from build123d import *

# Parameters (mm, degrees)
F0_W     = 3.9
F0_H     = 3.5
F1_DEPTH = 0.7
F3_DEPTH = 1
F4_SIZE  = 0.3
F6_DEPTH = 0.7


with BuildPart() as f1:
    # F0 (on Right) → F1 (new body)
    with BuildSketch(Plane.YZ):
        Rectangle(F0_W, F0_H)
        with BuildLine():
            Line((-1.95, 1.75), (1.95, 1.75))
            ThreePointArc((1.95, 1.75), (0, 3.7), (-1.95, 1.75))
        make_face()
        with BuildLine():
            ThreePointArc((-1.95, -1.75), (0, -3.7), (1.95, -1.75))
            Line((1.95, -1.75), (-1.95, -1.75))
        make_face()
    extrude(amount=F1_DEPTH)

    # F2 (on face) → F3 (join)
    with BuildSketch(Plane.YZ.offset(0.7)):
        Polygon((1.05, 1.143782), (1.05, 2.356218), (0, 2.962436), (-1.05, 2.356218), (-1.05, 1.143782), (0, 0.537564), align=None)
    extrude(amount=F3_DEPTH)

    # F4
    f4_edges = [f1.edges().sort_by_distance(p)[0] for p in [
        (1.7, -0.525, 2.659327),
        (1.7, 0.525, 2.659327),
        (1.7, 1.05, 1.75),
        (1.7, 0.525, 0.840673),
        (1.7, -0.525, 0.840673),
        (1.7, -1.05, 1.75),
    ]]
    chamfer(f4_edges, length=F4_SIZE)

    # F5 (on face) → F6 (cut, through all)
    with BuildSketch(Plane(origin=(0, 0, 0), x_dir=(0, -1, 0), z_dir=(-1, 0, 0))):
        Polygon((1.1, -2.385085), (1.1, -1.114915), (0, -0.479829), (-1.1, -1.114915), (-1.1, -2.385085), (0, -3.020171), align=None)
    extrude(amount=-F6_DEPTH, mode=Mode.SUBTRACT)


solid = f1.part
Build history of the part. All positions in model axes, mm. A direction names the side the tool comes from. Round coordinates to 2 decimals unless told otherwise and drop trailing zeros. Write each loop counter-clockwise with the first axis right and the second up, starting at its lowest first coordinate (ties: lowest second). Pieces come first, ordered by that corner, then holes. Notation, with made-up numbers: (-16.5, 69) - (40.5, 69) arc R25 cw to (40.5, 103) - close; hole circle Ø4 at (80, 61). An arc over 180 degrees is marked (long way). One line per question, with ' | ' between items.
1. Band-saw the part on B-B, the plane y = 0.2. Write the cut outline in (x, z), and give its area (3 significant figures).
Results are:
outline: (0, -3.69) - (0.7, -3.69) - (0.7, -2.9) - (0, -2.9) - close; (0, -0.6) - (0.7, -0.6) - (0.7, 0.65) - (1.4, 0.65) - (1.7, 1) - (1.7, 2.5) - (1.4, 2.85) - (0.7, 2.85) - (0.7, 3.69) - (0, 3.69) - close | area: 5.64 mm^2
2. Tool access for faces 1 (the face through (0, 0, 0)), 2 (the face through (0.7, 0, 0)): list every direction of +Z, -Z, +X, -X, +Y, -Y with a clear straight run to the whole face (end or side of a thin tool).
Results are:
face 1: +Z, -Z, -X, +Y, -Y | face 2: +X
3. Band-saw the part on D-D, the plane z = -0.25. Write the cut outline in (x, y), and give its area (3 significant figures).
Results are:
outline: (0, -1.95) - (0.7, -1.95) - (0.7, 1.95) - (0, 1.95) - close | area: 2.73 mm^2
4. Drill centre lines: line 1 along Y through (x, z) = (0.6, -1.75); line 2 along X through (y, z) = (1.65, -0.5); line 3 along Y through (x, z) = (0.1, -0.75). Where is each one in solid material? Low to high. Write a range as from..to.
Results are:
line 1: -1.95..-1.1, 1.1..1.95 | line 2: 0..0.7 | line 3: -1.95..-0.47, 0.47..1.95
5. Band-saw the part on C-C, the plane z = 2.5. Write the cut outline in (x, y).
Results are:
outline: (0, -1.8) - (0.7, -1.8) - (0.7, -0.8) - (1.4, -0.8) - (1.7, -0.2) - (1.7, 0.2) - (1.4, 0.8) - (0.7, 0.8) - (0.7, 1.8) - (0, 1.8) - close
6. Drop a flat-ended pin along its axis: pin 1 Ø1 at (x, y) = (0, 1.5) entering from -Z. Give the stop position or say it passes through.
Results are:
pin 1: z = -3.42
7. Band-saw the part on A-A, the plane x = 1.3. Write the cut outline in (y, z), and give its area (3 significant figures).
Results are:
outline: (-1.05, 1.14) - (0, 0.54) - (1.05, 1.14) - (1.05, 2.36) - (0, 2.96) - (-1.05, 2.36) - close | area: 3.82 mm^2
